For this review, take the finished solid that the model builds, in its own axes (mm). A direction names the side the tool comes from. Round coordinates to 2 decimals unless told otherwise and drop trailing zeros. Write each loop counter-clockwise with the first axis right and the second up, starting at its lowest first coordinate (ties: lowest second). Pieces come first, ordered by that corner, then holes. Notation, with made-up numbers: (82, -19) - (96, -19) arc R20 ccw to (96, 6) - close; hole circle Ø10 at (70.25, 49). An arc over 180 degrees is marked (long way). Answer in a Markdown table with one row per item. Add a question column.
Autodesk Inventor part; units mm, degrees
ref_plane "YZ Plane" through (0, 0, 0) normal (1, 0, 0) x (0, 1, 0)
ref_plane "XZ Plane" through (0, 0, 0) normal (0, 1, 0) x (-1, 0, 0)
ref_plane "XY Plane" through (0, 0, 0) normal (0, 0, 1) x (1, 0, 0)
sketch "Skizze1" plane through (0, 0, 0) normal (0, 0, 1) x (1, 0, 0)
  line L0 (-18.1618, 0.375) -> (-21.3761, 7.875)
  line L1 (-2.9476, 7.875) -> (-6.1618, 0.375)
  line L2 (-6.1618, 0.375) -> (-18.1618, 0.375)
  line L3 (-18.1618, 0.375) -> (-31.1618, 0.375)
  line L4 (-31.1618, 0.375) -> (-31.1618, 11.375)
  line L5 (-31.1618, 11.375) -> (6.8382, 11.375)
  line L6 (6.8382, 11.375) -> (6.8382, 0.375)
  line L7 (6.8382, 0.375) -> (-6.1618, 0.375)
  line L8 (-21.5376, 7.875) -> (-2.9476, 7.875)
  point P0 (0, 0)
  point P1 (-21.1618, 7.375)
  point P2 (-3.1618, 7.375)
  dimension "d10" = 38
  dimension "d14" = 12
  dimension "d17" = 13
  dimension "d27" = 18.59
  dimension "d28" = 7.5
  dimension "d29" = 3.2143
  dimension "d30" = 3.2143
extrude "Extrusion1" add sketch "Skizze1" along normal blind 50 contours L3 L4 L5 L6 L7 L1 L8 L0
sketch "Skizze2" plane through (6.8382, 0.375, 0) normal (1, 0, 0) x (0, 0, -1)
  line L0 (-50, 0) -> (-50, 11)
  line L1 (0, 11) -> (-50, 11)
  point P0 (0, -0.375)
  point P1 (-25, 4.85)
  dimension "d19" = 6.15
hole "Bohrung1" at (6.8382, 5.225, 25) direction (-1, 0, 0) diameter 3.3 depth 13 tip angle 118
properties part number "Schienenläuderaufsatz_15.11."
Q1. Add section C-C on z = 34.5. State the section outline as (x, y) points (3 decimals), then the cut area to 3 significant figures.
Q2. Add section D-D on y = 2.5. State the section outline as (x, z) points.
Q3. Add section B-B on y = 6. State the section outline as (x, z) points, then the cut area to 3 significant figures.
Q4. Tool access review of faces 1 (the face through (-12, 7.875, 25)), 2 (the face through (0.94, 3.59, 25.21)), 3 (the face through (6.838, 7.2, 24.6)): name each direction out of +Z, -Z, +X, -X, +Y, -Y from which nothing blocks a thin tool from reaching the whole face with its end or side.
Q5. To check wall thickness, follow probe 1 along Y at (x, z) = (4, 25) (3 decimals); probe 2 along Y at (x, z) = (-14.5, 12) (3 decimals); probe 3 along X at (y, z) = (3.5, 4). State the ranges of each line that lie inside material, in increasing order.
Q6. Draft analysis for pull direction X (two halves, no side actions). For faces 4 (the face through (-4.89, 3.34, 24.65)), 5 (the face through (-31.162, 6, 25)), 6 (the face through (-25, 0.375, 25)), state which applies: released by +X, released by -X, zero draft, split by the parting line, or undercut.
Q7. Add section A-A on z = 24. State the section outline as (x, y) points (3 decimals).
Answer sheet:
| question | item | result |
|---|---|---|
| 1 | outline | (-31.162, 0.375) - (-18.162, 0.375) - (-21.376, 7.875) - (-2.948, 7.875) - (-6.162, 0.375) - (6.838, 0.375) - (6.838, 11.375) - (-31.162, 11.375) - close |
| 1 | area | 304 mm² |
| 2 | outline | (-31.16, 0) - (-19.07, 0) - (-19.07, 50) - (-31.16, 50) - close; (-5.25, 0) - (6.84, 0) - (6.84, 50) - (-5.25, 50) - close |
| 3 | outline | (-31.16, 0) - (-20.57, 0) - (-20.57, 50) - (-31.16, 50) - close; (-3.75, 0) - (6.84, 0) - (6.84, 23.54) - (-3.75, 23.54) - close; (-3.75, 26.46) - (6.84, 26.46) - (6.84, 50) - (-3.75, 50) - close |
| 3 | area | 1,030 mm² |
| 4 | face 1 | +Z, -Z |
| 4 | face 2 | +X |
| 4 | face 3 | +Z, -Z, +X, +Y, -Y |
| 5 | probe 1 | y = 0.375 to 3.575, 6.875 to 11.375 |
| 5 | probe 2 | y = 7.875 to 11.375 |
| 5 | probe 3 | x = -31.16 to -19.5, -4.82 to 6.84 |
| 6 | face 4 | undercut |
| 6 | face 5 | released by -X |
| 6 | face 6 | zero draft |
| 7 | outline | (-31.162, 0.375) - (-18.162, 0.375) - (-21.376, 7.875) - (-2.948, 7.875) - (-3.521, 6.537) - (6.838, 6.537) - (6.838, 11.375) - (-31.162, 11.375) - close; (-6.162, 0.375) - (6.838, 0.375) - (6.838, 3.913) - (-4.646, 3.913) - close |
